The figure shows three views and two pictorial views of one solid part (mm, origin at its lowest corner). Answer the questions. A direction names the side the tool comes from. Round coordinates to 2 decimals unless told otherwise and drop trailing zeros. Order: outer loops, then holes, each group sorted by start corner. A loop starts at its lowest first (then second) coordinate and runs counter-clockwise, first axis right, second up. Notation, with made-up numbers: M -6.75,-17 L 30.25,-17 A31 ccw 30.25,22 Z; hole C 42,9.25 d6. An arc over 180 degrees is marked long. Answer as CSV lines item,"result".
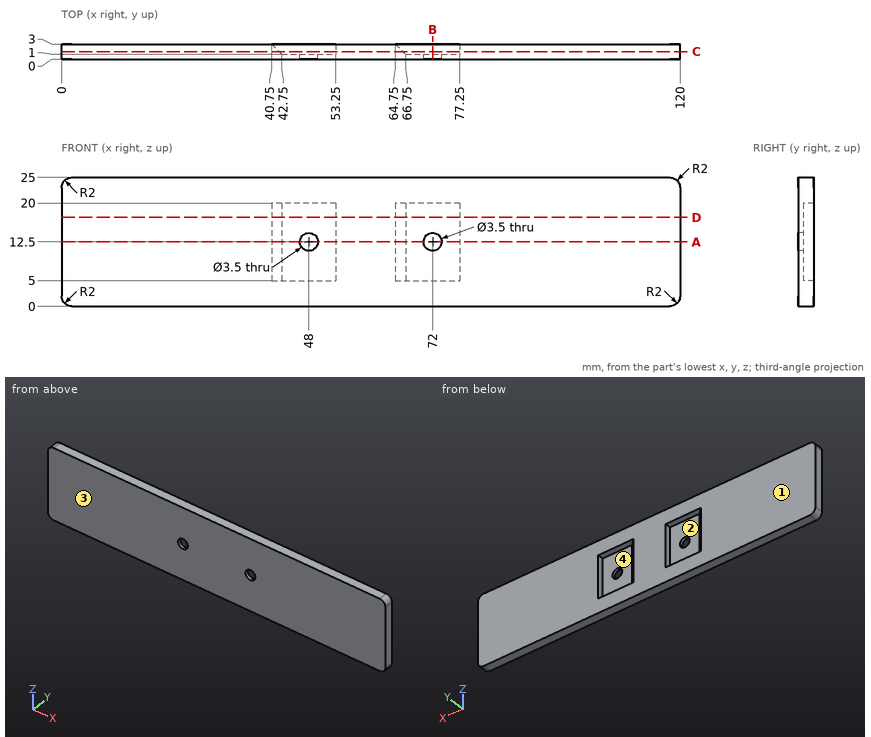
Item 1: A cutting plane is placed at B-B, the plane x = 72. Determine the outline of the cut face in (y, z).
Ans:
outline,"M 0,0 L 3,0 L 3,5 L 1,5 L 1,10.75 L 0,10.75 Z; M 0,14.25 L 1,14.25 L 1,20 L 3,20 L 3,25 L 0,25 Z"
Item 2: A tool of negligible diameter and unlimited length cuts with its end or side. For the marked faces 1 and 2, from which of +Z, -Z, +X, -X, +Y, -Y can it reach the whole face along a straight path? Write none if from no direction.
Ans:
face 1,"+Z, -Z, +X, -X, +Y"
face 2,"+Y"
Item 3: A cutting plane is placed at D-D, the plane z = 17.25. Determine the outline of the cut face in (x, y).
Ans:
outline,"M 0,0 L 120,0 L 120,3 L 77.25,3 L 77.25,1 L 66.75,1 L 64.75,3 L 53.25,3 L 53.25,1 L 42.75,1 L 40.75,3 L 0,3 Z"
Item 4: A cutting plane is placed at A-A, the plane z = 12.5. Determine the outline of the cut face in (x, y), and give its area (3 significant figures).
Ans:
outline,"M 0,0 L 46.25,0 L 46.25,1 L 42.75,1 L 40.75,3 L 0,3 Z; M 49.75,0 L 70.25,0 L 70.25,1 L 66.75,1 L 64.75,3 L 53.25,3 L 53.25,1 L 49.75,1 Z; M 73.75,0 L 120,0 L 120,3 L 77.25,3 L 77.25,1 L 73.75,1 Z"
area,"307 mm2"
Item 5: A cutting plane is placed at C-C, the plane y = 1.5. Determine the outline of the cut face in (x, z), and give its area (3 significant figures).
Ans:
outline,"M 0,2 A2 ccw 2,0 L 118,0 A2 ccw 120,2 L 120,23 A2 ccw 118,25 L 2,25 A2 ccw 0,23 Z; hole M 42.25,5 L 53.25,5 L 53.25,20 L 42.25,20 Z; hole M 66.25,5 L 77.25,5 L 77.25,20 L 66.25,20 Z"
area,"2,670 mm2"
Item 6: Find the intervals of material crossed by probe 1 along X at (y, z) = (0.5, 12.5); probe 2 along Z at (x, y) = (72, 0.25); probe 3 along X at (y, z) = (1.35, 19.25), in increasing order. Write a range as [from, to].
Ans:
probe 1,"[0, 46.25], [49.75, 70.25], [73.75, 120]"
probe 2,"[0, 10.75], [14.25, 25]"
probe 3,"[0, 42.4], [53.25, 66.4], [77.25, 120]"
Item 7: Determine the mould class of the marked faces 3 and 4 for opening direction X: +X half, -X half, draft (parallel to the pull), parting line (faces both ways), or undercut.
Ans:
face 3,"draft"
face 4,"undercut"
